Verification items for this drawing (mm, ordinates from the low corner). A direction names the side the tool comes from. Round coordinates to 2 decimals unless told otherwise and drop trailing zeros. Loops run counter-clockwise (first coordinate to the right, second up) from the corner with the lowest first, then second, coordinate; pieces in that order, holes last. Notation, with made-up numbers: M -17.5,79.25 L -13.5,79.25 A20 cw -13.5,116.25 Z; hole C 3,65.5 d11. An arc over 180 degrees is marked long. Answer as CSV lines item,"result".
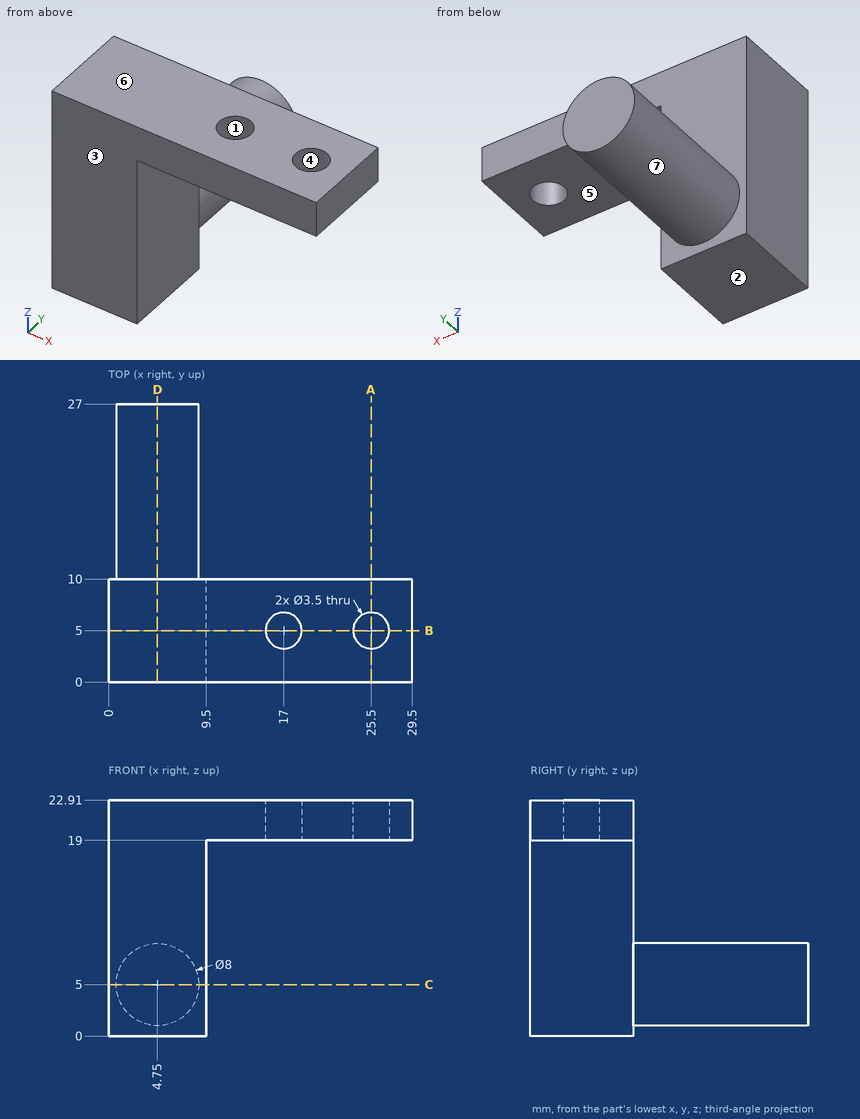
1) Material ranges on probe 1 along Y at (x, z) = (25.5, 20.9); probe 2 along Z at (x, y) = (10.5, 4.75); probe 3 along X at (y, z) = (4, 3), recorded low to high.
Here are the results:
probe 1,"y = 0 to 3.25, 6.75 to 10"
probe 2,"z = 19 to 22.91"
probe 3,"x = 0 to 9.5"
2) Section check D-D (x = 4.75). Record the cut outline in (y, z).
Here are the results:
outline,"M 0,0 L 10,0 L 10,1 L 27,1 L 27,9 L 10,9 L 10,22.91 L 0,22.91 Z"
3) Section check C-C (z = 5). Record the cut outline in (x, y), plus the area to 3 significant figures.
Here are the results:
outline,"M 0,0 L 9.5,0 L 9.5,10 L 8.75,10 L 8.75,27 L 0.75,27 L 0.75,10 L 0,10 Z"
area,"231 mm^2"
4) Section check A-A (x = 25.5). Record the cut outline in (y, z), plus the area to 3 significant figures.
Here are the results:
outline,"M 0,19 L 3.25,19 L 3.25,22.91 L 0,22.91 Z; M 6.75,19 L 10,19 L 10,22.91 L 6.75,22.91 Z"
area,"25.4 mm^2"
5) Draft check along Y on the marked faces 1, 2, 3 and 4. Enter one of: +Y half, -Y half, draft (parallel to the pull), parting line (faces both ways), or undercut.
Here are the results:
face 1,"undercut"
face 2,"draft"
face 3,"-Y half"
face 4,"undercut"
6) Section check B-B (y = 5). Record the cut outline in (x, z).
Here are the results:
outline,"M 0,0 L 9.5,0 L 9.5,19 L 15.25,19 L 15.25,22.91 L 0,22.91 Z; M 18.75,19 L 23.75,19 L 23.75,22.91 L 18.75,22.91 Z; M 27.25,19 L 29.5,19 L 29.5,22.91 L 27.25,22.91 Z"
7) Set-up check for the marked faces 5, 6 and 7: record each of +Z, -Z, +X, -X, +Y, -Y from which the full face is reachable in a straight line by a thin tool's end or side.
Here are the results:
face 5,"-Z, +X, +Y, -Y"
face 6,"+Z, +X, -X, +Y, -Y"
face 7,"+Y"
8) Go/stop test with flat-tipped pins: pin 1 (4.5 mm diameter, centred on x = 25.5, y = 5, fed in from -Z); pin 2 (12 mm diameter, centred on y = 21, z = 14, fed in from +X); pin 3 (6 mm diameter, centred on x = 6, y = 18, fed in from -Z). Record where each tip stops, or that it passes through.
Here are the results:
pin 1,"stops at z = 19"
pin 2,"stops at x = 7.4"
pin 3,"stops at z = 1"
